from build123d import *

# Parameters (mm, degrees)
SKETCH002_W         = 117
SKETCH002_H         = 138
PAD001_DEPTH        = 4
SKETCH003_R         = 3
PAD002_DEPTH        = 10
SKETCH004_R         = 1
POCKET_DEPTH        = 0.001
POCKET_DEPTH_BACK   = 10.001
PAD003_DEPTH        = 50
PAD004_DEPTH        = 8
LINEARPATTERN_COUNT = 2
LINEARPATTERN_PITCH = 80
SKETCH007_R         = 1
POCKET001_DEPTH     = 10
SKETCH008_R         = 1.85
POCKET002_DEPTH     = 7


with BuildPart() as part:
    # Sketch002 → Pad001 (new body)
    with BuildSketch(Plane.XY):
        with Locations((0, 30)):
            Rectangle(SKETCH002_W, SKETCH002_H)
    extrude(amount=PAD001_DEPTH)

    # Sketch003 → Pad002 (join)
    with BuildSketch(Plane.XY):
        with Locations((43.5, -29)):
            Circle(SKETCH003_R)
        with Locations((43.5, 29)):
            Circle(SKETCH003_R)
        with Locations((-43.5, 29)):
            Circle(SKETCH003_R)
        with Locations((-43.5, -29)):
            Circle(SKETCH003_R)
    extrude(amount=PAD002_DEPTH)

    # Sketch004 → Pocket (cut, two sides)
    with BuildSketch(Plane.XY) as pocket_sk:
        with Locations((43.5, -29)):
            Circle(SKETCH004_R)
        with Locations((43.5, 29)):
            Circle(SKETCH004_R)
        with Locations((-43.5, 29)):
            Circle(SKETCH004_R)
        with Locations((-43.5, -29)):
            Circle(SKETCH004_R)
    extrude(amount=-POCKET_DEPTH, mode=Mode.SUBTRACT)
    extrude(pocket_sk.sketch, amount=POCKET_DEPTH_BACK, mode=Mode.SUBTRACT)

    # Sketch005 → Pad003 (join)
    with BuildSketch(Plane.XY):
        Polygon((-59, -40), (59, -40), (59, 99), (55, 99), (55, -36), (-55, -36), (-55, 99), (-59, 99), align=None)
    extrude(amount=PAD003_DEPTH)

    # Sketch006 → Pad004 (join)
    with BuildSketch(Plane(origin=(0, -36, 0), x_dir=(-1, 0, 0), z_dir=(0, 1, 0))):
        Polygon((-55, 50), (-55, 42), (-47, 50), align=None)
        Polygon((47, 50), (55, 42), (55, 50), align=None)
    pad004 = extrude(amount=PAD004_DEPTH)

    # LinearPattern: Pad004 ×2
    with Locations(*[(0, i * LINEARPATTERN_PITCH, 0) for i in range(1, LINEARPATTERN_COUNT)]):
        add(pad004)

    # Sketch007 → Pocket001 (cut)
    with BuildSketch(Plane.XY.offset(50)):
        with Locations((52, -32)):
            Circle(SKETCH007_R)
        with Locations((-52, -32)):
            Circle(SKETCH007_R)
        with Locations((-52, 48)):
            Circle(SKETCH007_R)
        with Locations((52, 48)):
            Circle(SKETCH007_R)
    extrude(amount=-POCKET001_DEPTH, mode=Mode.SUBTRACT)

    # Sketch008 → Pocket002 (cut)
    with BuildSketch(Plane.YZ.offset(59)):
        with Locations((-24, 15)):
            Circle(SKETCH008_R)
        with Locations((30, 15)):
            Circle(SKETCH008_R)
        with Locations((30, 46)):
            Circle(SKETCH008_R)
        with Locations((-24, 46)):
            Circle(SKETCH008_R)
    extrude(amount=-POCKET002_DEPTH, mode=Mode.SUBTRACT)


solid = part.part
Read the model definition and answer for the solid it produces. Units are mm, in the model's axes. A direction names the side the tool comes from. Coordinates: 2 decimals unless noted, no trailing zeros. Loops run counter-clockwise (first coordinate to the right, second up) from the corner with the lowest first, then second, coordinate; pieces in that order, holes last. Notation, with made-up numbers: (-24.75, 12) -> (-17.75, 12) arc R23 cw to (-17.75, 20) -> close; hole circle Ø8 at (70.5, 26). An arc over 180 degrees is marked (long way). Answer in a Markdown table with one row per item.
Item 1: A cutting plane is placed at B-B on y = -24. Determine the outline of the cut face in (x, z), plus the area to 3 significant figures.
Returned:
| item | result |
|---|---|
| outline | (-59, 0) -> (59, 0) -> (59, 13.15) -> (55, 13.15) -> (55, 4) -> (-55, 4) -> (-55, 50) -> (-59, 50) -> close; (55, 16.85) -> (59, 16.85) -> (59, 44.15) -> (55, 44.15) -> close; (55, 47.85) -> (59, 47.85) -> (59, 50) -> (55, 50) -> close |
| area | 810 mm^2 |
Item 2: A cutting plane is placed at D-D on y = 62. Determine the outline of the cut face in (x, z).
Returned:
| item | result |
|---|---|
| outline | (-59, 0) -> (59, 0) -> (59, 50) -> (55, 50) -> (55, 4) -> (-55, 4) -> (-55, 50) -> (-59, 50) -> close |
Item 3: For faces 4 (the cylindrical face through (57.03, -25.85, 15.08)), 5 (the flat face through (45, -29, 10)), 6 (the cylindrical face through (-46.5, 29.1, 7)), 7 (the flat face through (-1, -40, 25)), 8 (the flat face through (5, 99, 3)), determine the directions among +Z, -Z, +X, -X, +Y, -Y from which every point of the face is accessible in a straight line to the end or side of a thin tool.
Returned:
| item | result |
|---|---|
| face 4 | +X |
| face 5 | +Z, +Y |
| face 6 | +Z |
| face 7 | +Z, -Z, +X, -X, -Y |
| face 8 | +Z, -Z, +X, -X, +Y |
Item 4: Each of these flat-tipped pins is pushed along its axis until it touches: P1, Ø5, axis at x = -44.5, y = 28.5, coming from the +Z side; P2, Ø8, axis at x = 36.5, y = -4.5, coming from the -Z side; P3, Ø1.2, axis at x = -52, y = 48, coming from the +Z side; P4, Ø4, axis at x = 52, z = 48, coming from the +Y side. Where does it stop, or does it pass through?
Returned:
| item | result |
|---|---|
| P1 | stops at z = 10 |
| P2 | stops at z = 0 |
| P3 | stops at z = 4 |
| P4 | stops at y = 52 |
Item 5: Straight lines are drawn through the part: line 1 along Z through (x, y) = (57, -24); line 2 along X through (y, z) = (29, 6); line 3 along X through (y, z) = (-33.5, 29). For each, find the intervals that lie inside material, in ascending order. Write a range as [from, to].
Returned:
| item | result |
|---|---|
| line 1 | z = [0, 13.15], [16.85, 44.15], [47.85, 50] |
| line 2 | x = [-59, -55], [-46.5, -44.5], [-42.5, -40.5], [40.5, 42.5], [44.5, 46.5], [55, 59] |
| line 3 | x = [-59, -55], [55, 59] |
Item 6: A cutting plane is placed at A-A on z = 36.5. Determine the outline of the cut face in (x, y).
Returned:
| item | result |
|---|---|
| outline | (-59, -40) -> (59, -40) -> (59, 99) -> (55, 99) -> (55, -36) -> (-55, -36) -> (-55, 99) -> (-59, 99) -> close |
Item 7: A cutting plane is placed at C-C on x = 22. Determine the outline of the cut face in (y, z).
Returned:
| item | result |
|---|---|
| outline | (-40, 0) -> (99, 0) -> (99, 4) -> (-36, 4) -> (-36, 50) -> (-40, 50) -> close |
Item 8: For a pull along X with two mould halves and no side action, classify faces 1 (the flat face through (59, 29, 25)), 2 (the flat face through (52, -28, 47)), 3 (the cylindrical face through (57.028, 28.532, 44.874)) as released by +X, released by -X, zero draft, split by the parting line, or undercut.
Returned:
| item | result |
|---|---|
| face 1 | released by +X |
| face 2 | undercut |
| face 3 | zero draft |
